Work out the finished part from the listing and answer in its coordinate system (mm). Face numbers are marked on the shaded views. A direction names the side the tool comes from. Round coordinates to 2 decimals unless told otherwise and drop trailing zeros. Order: outer loops, then holes, each group sorted by start corner. A loop starts at its lowest first (then second) coordinate and runs counter-clockwise, first axis right, second up. Notation, with made-up numbers: (-34, -4) -> (17, -4) arc R23 cw to (17, 10) -> close; hole circle Ø11 at (11.25, 61.5). An arc over 180 degrees is marked (long way). Use a Markdown table: item, result. Add a question column.
Item 1: A cutting plane is placed at B-B, the plane z = -1. Determine the outline of the cut face in (x, y) (3 decimals), plus the area to 3 significant figures.
Item 2: Find the intervals of material crossed by L1, parallel to Y at x = 3, z = 0.75; L2, parallel to Z at x = 0.75, y = 0.3; L3, parallel to X at y = -0.05, z = -0.75, in increasing order. Write a range as [from, to].
Item 3: A tool of negligible diameter and unlimited length cuts with its end or side. For the marked faces 1, 2 and 3, from which of +Z, -Z, +X, -X, +Y, -Y can it reach the whole face along a straight path? Write none if from no direction.
Item 4: A cutting plane is placed at A-A, the plane x = 0. Determine the outline of the cut face in (y, z).
Item 5: Flat-ended cylindrical pins translate along their axes: P1, Ø3, axis at x = -1.5, z = 1.5, coming from the +Y side; P2, Ø1.5, axis at x = 1, y = 1.5, coming from the -Z side; P3, Ø1.3, axis at x = 1, z = 1.5, coming from the -Y side. Find the tip coordinate at first contact, or state that the pin passes through.
Item 6: A cutting plane is placed at C-C, the plane y = 0. Determine the outline of the cut face in (x, z) (3 decimals), plus the area to 3 significant figures.
Item 7: A cutting plane is placed at D-D, the plane z = 2. Determine the outline of the cut face in (x, y) (3 decimals).
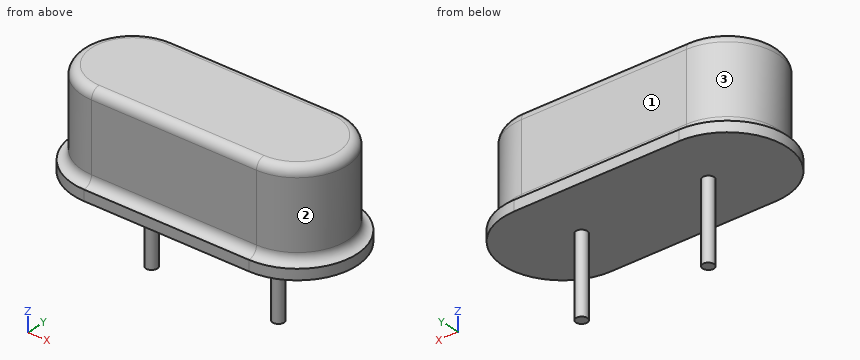
from build123d import *

# Parameters (mm, degrees)
BOSS_EXTRUDE1_DEPTH = 3.68
SKETCH4_R           = 0.215
BOSS_EXTRUDE2_DEPTH = 3


with BuildPart() as part:
    # Sketch1 → Boss-Extrude1 (new body)
    with BuildSketch(Plane.XY):
        with BuildLine():
            Line((-3.175, 2.25), (3.175, 2.25))
            ThreePointArc((3.175, 2.25), (5.425, 0), (3.175, -2.25))
            Line((3.175, -2.25), (-3.175, -2.25))
            ThreePointArc((-3.175, -2.25), (-5.425, 0), (-3.175, 2.25))
        make_face()
    extrude(amount=BOSS_EXTRUDE1_DEPTH)

    # Cut-Sweep1: sweep along a path in Sketch1_2
    with BuildLine(Plane.XY) as cut_sweep1_path:
        Line((-3.175, 2.25), (3.175, 2.25))
        ThreePointArc((3.175, 2.25), (5.425, 0), (3.175, -2.25))
        Line((3.175, -2.25), (-3.175, -2.25))
        ThreePointArc((-3.175, -2.25), (-5.425, 0), (-3.175, 2.25))
    # Sketch2 → Cut-Sweep1 (sweep, cut)
    with BuildSketch(Plane(origin=(0, 0, 0), x_dir=(0, 0, -1), z_dir=(1, 0, 0))):
        with BuildLine():
            Line((-0.75, 1.9), (-3.33, 1.9))
            ThreePointArc((-3.33, 1.9), (-3.577487373, 1.797487373), (-3.68, 1.55))
            Line((-3.68, 1.55), (-3.68, 2.25))
            Line((-3.68, 2.25), (-0.4, 2.25))
            ThreePointArc((-0.4, 2.25), (-0.502512627, 2.002512627), (-0.75, 1.9))
        make_face()
    sweep(path=cut_sweep1_path.line, mode=Mode.SUBTRACT)

    # Sketch4 → Boss-Extrude2 (add)
    with BuildSketch(Plane(origin=(0, 0, 0), x_dir=(-1, 0, 0), z_dir=(0, 0, -1))):
        with Locations(Location((-2.44, 0, 0), (0, 0, 180))):
            Circle(SKETCH4_R)
        with Locations(Location((2.44, 0, 0), (0, 0, 180))):
            Circle(SKETCH4_R)
    extrude(amount=BOSS_EXTRUDE2_DEPTH)


solid = part.part
Reported:
| question | item | result |
|---|---|---|
| 1 | outline | circle Ø0.43 at (-2.44, 0); circle Ø0.43 at (2.44, 0) |
| 1 | area | 0.290 mm² |
| 2 | L1 | [-1.9, 1.9] |
| 2 | L2 | [0, 3.68] |
| 2 | L3 | [-2.65, -2.23], [2.23, 2.65] |
| 3 | face 1 | +Z, +X, -X, +Y |
| 3 | face 2 | +Z, +X |
| 3 | face 3 | +Z, -X |
| 4 | outline | (-2.25, 0) -> (2.25, 0) -> (2.25, 0.4) arc R0.35 cw to (1.9, 0.75) -> (1.9, 3.33) arc R0.35 ccw to (1.55, 3.68) -> (-1.55, 3.68) arc R0.35 ccw to (-1.9, 3.33) -> (-1.9, 0.75) arc R0.35 cw to (-2.25, 0.4) -> close |
| 5 | P1 | y = 2.25 |
| 5 | P2 | z = 0 |
| 5 | P3 | y = -1.9 |
| 6 | outline | (-5.425, 0) -> (-2.655, 0) -> (-2.655, -3) -> (-2.225, -3) -> (-2.225, 0) -> (2.225, 0) -> (2.225, -3) -> (2.655, -3) -> (2.655, 0) -> (5.425, 0) -> (5.425, 0.4) arc R0.35 cw to (5.075, 0.75) -> (5.075, 3.33) arc R0.35 ccw to (4.725, 3.68) -> (-4.725, 3.68) arc R0.35 ccw to (-5.075, 3.33) -> (-5.075, 0.75) arc R0.35 cw to (-5.425, 0.4) -> close |
| 6 | area | 40.2 mm² |
| 7 | outline | (-3.175, -1.9) -> (3.175, -1.9) arc R1.9 ccw to (3.175, 1.9) -> (-3.175, 1.9) arc R1.9 ccw to start |
